The model under review builds one solid part; all positions refer to its coordinate system, in mm. Face numbers are marked on the shaded views. A direction names the side the tool comes from. Round coordinates to 2 decimals unless told otherwise and drop trailing zeros. Order: outer loops, then holes, each group sorted by start corner. A loop starts at its lowest first (then second) coordinate and runs counter-clockwise, first axis right, second up.
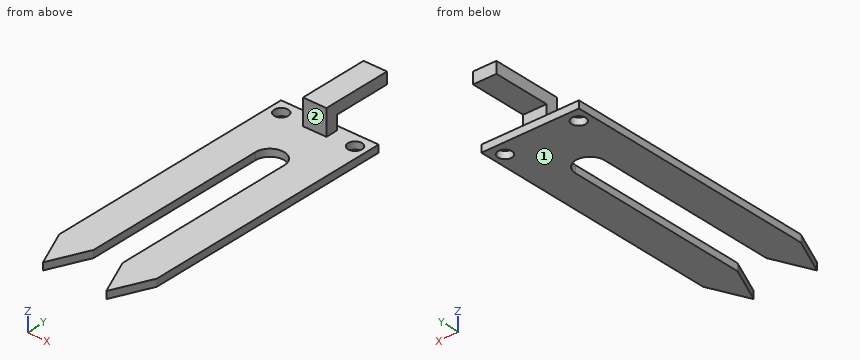
Autodesk Inventor part; units mm, degrees
ref_plane "YZ Plane" through (0, 0, 0) normal (1, 0, 0) x (0, 1, 0)
ref_plane "XZ Plane" through (0, 0, 0) normal (0, 1, 0) x (-1, 0, 0)
ref_plane "XY Plane" through (0, 0, 0) normal (0, 0, 1) x (1, 0, 0)
sketch "Sketch1" plane through (0, 0, 0) normal (0, 0, 1) x (1, 0, 0)
  line L0 (-10.125, -30.55) -> (10.125, -30.55) construction
  line L1 (10.125, -30.55) -> (10.125, 30.55) construction
  line L2 (10.125, 30.55) -> (-10.125, 30.55)
  line L3 (-10.125, 30.55) -> (-10.125, -30.55) construction
  line L4 (-10.125, -30.55) -> (10.125, 30.55) construction
  line L5 (10.125, -30.55) -> (-10.125, 30.55) construction
  line L6 (-10.125, 30.55) -> (-10.125, -22.55)
  line L7 (-10.125, -22.55) -> (-6.56, -30.55)
  line L8 (-6.56, -30.55) -> (-2.995, -22.55)
  line L9 (-2.995, -22.55) -> (-2.995, 16.2)
  arc A0 (2.995, 16.2) -> (-2.995, 16.2) centre (0, 16.2) ccw
  line L10 (0, 0) -> (0, 8.9972) construction
  line L11 (10.125, 30.55) -> (10.125, -30.55) construction
  line L12 (10.125, 30.55) -> (10.125, -22.55)
  line L13 (10.125, -22.55) -> (6.56, -30.55)
  line L14 (6.56, -30.55) -> (2.995, -22.55)
  line L15 (2.995, -22.55) -> (2.995, 16.2)
  dimension "d0" = 20.25
  dimension "d1" = 61.1
  dimension "d2" = 8
  dimension "d3" = 3.565
  dimension "d4" = 14.35
extrude "Extrusion1" add sketch "Sketch1" along normal blind 1.5
sketch "Sketch2" plane through (0, 0, 1.5) normal (0, 0, 1) x (1, 0, 0)
  line L0 (-2.43, 29.43) -> (2.43, 29.43)
  line L1 (2.43, 29.43) -> (2.43, 26.93)
  line L2 (2.43, 26.93) -> (-2.43, 26.93)
  line L3 (-2.43, 26.93) -> (-2.43, 29.43)
  line L4 (-2.43, 29.43) -> (2.43, 26.93) construction
  line L5 (2.43, 29.43) -> (-2.43, 26.93) construction
  line L6 (10.125, 30.55) -> (-10.125, 30.55)
  point P0 (0, 0)
  point P1 (0, 28.18)
  dimension "d7" = 4.86
  dimension "d8" = 2.5
  dimension "d9" = 1.12
extrude "Extrusion2" add sketch "Sketch2" along normal blind 5.3
sketch "Sketch3" plane through (-2.43, 29.43, 1.5) normal (0, 1, 0) x (1, 0, 0)
  line L0 (0, 0) -> (0, -5.3)
  line L1 (0, -5.3) -> (4.86, -5.3)
  line L2 (4.86, -5.3) -> (4.86, -2.91)
  line L3 (4.86, -2.91) -> (0, -2.91)
  line L4 (0, -2.91) -> (0, -5.3)
  line L5 (4.86, 0) -> (4.86, -5.3)
  point P0 (2.43, 1.5)
  dimension "d12" = 2.39
extrude "Extrusion3" add sketch "Sketch3" along normal blind 12
sketch "Sketch4" plane through (0, 0, 1.5) normal (0, 0, 1) x (1, 0, 0)
  line L0 (-7.65, 27.75) -> (7.65, 27.75) construction
  circle A0 centre (-7.65, 27.75) radius 1.45
  circle A1 centre (7.65, 27.75) radius 1.45
  line L1 (10.125, 30.55) -> (-10.125, 30.55)
  point P0 (0, 0)
  point P1 (0, 27.75)
  point P2 (-7.65, 29.2)
  point P3 (-6.2, 27.75)
  point P4 (6.2, 27.75)
  dimension "d15" = 2.9
  dimension "d16" = 12.4
  dimension "d17" = 1.35
extrude "Extrusion4" cut sketch "Sketch4" against normal through all
properties part number "moist probe"
(1) To check wall thickness, follow probe 1 along X at (y, z) = (-18.5, 0.5) (3 decimals); probe 2 along Y at (x, z) = (-0.25, 0.5); probe 3 along Z at (x, y) = (-8.75, -1). State the ranges of each line that lie inside material, in increasing order.
Data:
probe 1: x = -10.125 to -2.995, 2.995 to 10.125
probe 2: y = 19.18 to 30.55
probe 3: z = 0 to 1.5
(2) Consider section B-B (x = -7.65). Write out the cut boundary in (y, z).
Data:
outline: (-28.1, 0) - (26.3, 0) - (26.3, 1.5) - (-28.1, 1.5) - close; (29.2, 0) - (30.55, 0) - (30.55, 1.5) - (29.2, 1.5) - close
(3) Consider section D-D (x = 0). Write out the cut boundary in (y, z) (3 decimals), and give its area (3 significant figures).
Data:
outline: (19.195, 0) - (30.55, 0) - (30.55, 1.5) - (29.43, 1.5) - (29.43, 4.41) - (41.43, 4.41) - (41.43, 6.8) - (26.93, 6.8) - (26.93, 1.5) - (19.195, 1.5) - close
area: 59.0 mm2
(4) Consider section A-A (y = -18). Write out the cut boundary in (x, z) (3 decimals).
Data:
outline: (-10.125, 0) - (-2.995, 0) - (-2.995, 1.5) - (-10.125, 1.5) - close; (2.995, 0) - (10.125, 0) - (10.125, 1.5) - (2.995, 1.5) - close
(5) Insertion check: pin 1 (2.5 mm diameter, centred on x = -0.5, z = 3, fed in from +Y); pin 2 (4 mm diameter, centred on y = 34, z = 4.5, fed in from -X); pin 3 (2.5 mm diameter, centred on x = 0.5, y = 33, fed in from -Z); pin 4 (4 mm diameter, centred on x = 8, z = 4, fed in from -Y). Each pin has a flat end and moves straight along its axis. Give the tip position at first contact, or say it passes through.
Data:
pin 1: stops at y = 29.43
pin 2: stops at x = -2.43
pin 3: stops at z = 4.41
pin 4: passes through
(6) Consider section C-C (y = 27.75). Write out the cut boundary in (x, z) (3 decimals), and give its area (3 significant figures).
Data:
outline: (-10.125, 0) - (-9.1, 0) - (-9.1, 1.5) - (-10.125, 1.5) - close; (-6.2, 0) - (6.2, 0) - (6.2, 1.5) - (2.43, 1.5) - (2.43, 6.8) - (-2.43, 6.8) - (-2.43, 1.5) - (-6.2, 1.5) - close; (9.1, 0) - (10.125, 0) - (10.125, 1.5) - (9.1, 1.5) - close
area: 47.4 mm2
(7) For the marked faces 1 and 2, list the 3-axis set-ups (+Z, -Z, +X, -X, +Y, -Y) from which the entire face can be reached by the end or side of a thin tool; tool diameter is ignored.
Data:
face 1: -Z, +X, -X, +Y, -Y
face 2: +Z, +X, -X, -Y
